Design review of the part built by this model. Coordinates are the model's own, in mm. A direction names the side the tool comes from. Give positions to 0.01 mm unless a question says otherwise; leave off trailing zeros. Loops run counter-clockwise (first coordinate to the right, second up) from the corner with the lowest first, then second, coordinate; pieces in that order, holes last. Notation, with made-up numbers: (-30.5, 26) -> (22.5, 26) arc R15 ccw to (22.5, 35) -> close; hole circle Ø8 at (-20, 89). An arc over 180 degrees is marked (long way). Answer in a Markdown table with one row per item. Add a question column.
(1) For pin 1 (5.5 mm diameter, centred on x = 0, y = -7.94, fed in from -Z); pin 2 (0.6 mm diameter, centred on y = -10.5, z = 7, fed in from -X); pin 3 (8 mm diameter, centred on y = -9, z = 21, fed in from +X); pin 4 (5 mm diameter, centred on y = -14, z = 14.5, fed in from -X), all flat-tipped, find the tip position at first contact; note any pin that passes through.
(2) For faces 4 (the cylindrical face through (188.908, -8.147, 47.841)), 5 (the flat face through (62, -8, 14.351)), 6 (the flat face through (173, -8, 12.7)), list the 3-axis set-ups (+Z, -Z, +X, -X, +Y, -Y) from which the entire face can be reached by the end or side of a thin tool; tool diameter is ignored.
(3) Draft analysis for pull direction X (two halves, no side actions). For faces 1 (the flat face through (62, -8, 39.751)), 2 (the flat face through (153.987, -8, 27)), 3 (the cylindrical face through (188.908, -8.147, 6.439)), state which applies: +X half, -X half, draft (parallel to the pull), parting line (faces both ways), or undercut.
(4) Consider section C-C on x = 81. Write out the cut boundary in (y, z) (3 decimals).
(5) For line 1 (Z direction, x = 170, y = -1.25); line 2 (Z direction, x = 124, y = -5); line 3 (Y direction, x = 181, z = 6) (3 decimals), list the stretches that pass through material, from the lowest coordinate up.
(6) Consider section A-A on y = -6. Count the separate pieces of the cut face and the enclosed holes in it, then the cut area to 3 significant figures.
(7) Consider section B-B on z = 25.5. Write out the cut boundary in (x, y) (1 decimal).
from build123d import *

# Parameters (mm, degrees)
F1_DEPTH = 54.102
F2_D     = 9.525
F3_W     = 25.4
F3_H     = 28.702
F3_W_2   = 38.1
F4_DEPTH = 25.4
F5_R     = 6.604
F6_W     = 141.2875
F6_H     = 14.351
F6_W_2   = 7.9375
F7_DEPTH = 25.4
F9_R     = 6.604


# Not quite as in the source:
# - a pattern or mirror of a feature is missing from the dataset's text; its kind, count and spacing are read off the source's solid


with BuildPart() as f1:
    # F0 (on Top) → F1 (new body)
    with BuildSketch(Plane.XY):
        with BuildLine():
            ThreePointArc((192.0875, -7.9375), (189.7626600757, -2.3248399243), (184.15, 0))
            Line((184.15, 0), (184.15, -15.875))
            ThreePointArc((184.15, -15.875), (189.7626600757, -13.5501600757), (192.0875, -7.9375))
        make_face()
        with BuildLine():
            Line((184.15, -15.875), (184.15, 0))
            ThreePointArc((184.15, 0), (176.2125, -7.9375), (184.15, -15.875))
        make_face()
        with BuildLine():
            Line((184.15, 0), (0, 0))
            ThreePointArc((0, 0), (5.6126600757, -2.3248399243), (7.9375, -7.9375))
            ThreePointArc((7.9375, -7.9375), (5.6126600757, -13.5501600757), (0, -15.875))
            Line((0, -15.875), (184.15, -15.875))
            ThreePointArc((184.15, -15.875), (176.2125, -7.9375), (184.15, 0))
        make_face()
        with BuildLine():
            ThreePointArc((7.9375, -7.9375), (5.6126600757, -2.3248399243), (0, 0))
            Line((0, 0), (0, -15.875))
            ThreePointArc((0, -15.875), (5.6126600757, -13.5501600757), (7.9375, -7.9375))
        make_face()
        with BuildLine():
            Line((0, -15.875), (0, 0))
            ThreePointArc((0, 0), (-7.9375, -7.9375), (0, -15.875))
        make_face()
    extrude(amount=F1_DEPTH)

    # F2 (through all)
    with Locations(Plane(origin=(0, 0, 0), x_dir=(1, 0, 0), z_dir=(0, 0, -1))):
        with Locations((0, 7.9375), (184.15, 7.9375)):
            Hole(F2_D / 2)

    # F3 (on Front) → F4 (cut)
    with BuildSketch(Plane.XZ):
        with Locations((204.7875, 27.051)):
            Rectangle(F3_W, F3_H)
        with Locations((173.0375, 27.051)):
            Rectangle(F3_W_2, F3_H)
    extrude(amount=F4_DEPTH, mode=Mode.SUBTRACT)

    # F5
    f5_edges = [f1.edges().sort_by_distance(p)[0] for p in [
        (153.9875, -7.9375, 41.402),
        (153.9875, -7.9375, 12.7),
    ]]
    fillet(f5_edges, radius=F5_R)

    # F6 (on Front) → F7 (cut)
    with BuildSketch(Plane.XZ):
        with Locations((70.64375, 46.9265)):
            Rectangle(F6_W, F6_H)
        with Locations((-3.96875, 46.9265)):
            Rectangle(F6_W_2, F6_H)
        Polygon((-20.6375, 39.751), (-7.9375, 39.751), (-7.9375, 54.102), (0, 54.102), (141.2875, 54.102), (141.2875, 66.802), (-20.6375, 66.802), align=None)
    f7 = extrude(amount=F7_DEPTH, mode=Mode.SUBTRACT)

    # F7_copies: F7 across plane
    add(f7.mirror(Plane(origin=(0, 0, 27.051), x_dir=(-1, 0, 0), z_dir=(0, 0, -1))), mode=Mode.SUBTRACT)

    # F9
    f9_edges = [f1.edges().sort_by_distance(p)[0] for p in [
        (141.2875, -7.9375, 39.751),
        (141.2875, -7.9375, 54.102),
        (141.2875, -7.9375, 0),
        (141.2875, -7.9375, 14.351),
    ]]
    fillet(f9_edges, radius=F9_R)


solid = f1.part
Values follow:
| question | item | result |
|---|---|---|
| 1 | pin 1 | through |
| 1 | pin 2 | x = 141.29 |
| 1 | pin 3 | x = 154.4 |
| 1 | pin 4 | x = -7.09 |
| 2 | face 4 | +Z, -Z |
| 2 | face 5 | -Z, -X, +Y, -Y |
| 2 | face 6 | +X, +Y, -Y |
| 3 | face 1 | draft |
| 3 | face 2 | +X half |
| 3 | face 3 | undercut |
| 4 | outline | (-15.875, 14.351) -> (0, 14.351) -> (0, 39.751) -> (-15.875, 39.751) -> close |
| 5 | line 1 | 0 to 12.7, 41.4 to 54.1 |
| 5 | line 2 | 14.35 to 39.75 |
| 5 | line 3 | -15.875 to -11.509, -4.366 to 0 |
| 6 | separate pieces | 4 |
| 6 | enclosed holes | 0 |
| 6 | area | 5,010 mm2 |
| 7 | outline | (0, -15.9) -> (154, -15.9) -> (154, 0) -> (0, 0) arc R7.9 ccw to start; hole circle Ø9.5 at (0, -7.9) |
